Autodesk Inventor part; units mm, degrees
ref_plane "YZ Plane" through (0, 0, 0) normal (1, 0, 0) x (0, 1, 0)
ref_plane "XZ Plane" through (0, 0, 0) normal (0, 1, 0) x (-1, 0, 0)
ref_plane "XY Plane" through (0, 0, 0) normal (0, 0, 1) x (1, 0, 0)
sketch "Sketch1" plane through (0, 0, 0) normal (0, 0, 1) x (1, 0, 0)
  line L0 (-22.1112, 10.3171) -> (130.2888, 10.3171)
  line L1 (130.2888, 10.3171) -> (130.2888, -65.8829)
  line L2 (130.2888, -65.8829) -> (-22.1112, -65.8829)
  line L3 (-22.1112, -65.8829) -> (-22.1112, 10.3171)
  point P0 (0, 0)
  dimension "d0" = 152.4
  dimension "d1" = 76.2
extrude "Extrusion1" add sketch "Sketch1" along normal blind 3.175
sketch "Sketch2" plane through (0, 0, 3.175) normal (0, 0, 1) x (1, 0, 0)
  circle A0 centre (-10.0607, -27.9271) radius 1.85
  circle A1 centre (6.0853, -27.9271) radius 1.85
  circle A2 centre (22.2313, -27.9271) radius 1.85
  circle A3 centre (38.3773, -27.9271) radius 1.85
  circle A4 centre (54.5233, -27.9271) radius 1.85
  circle A5 centre (70.6693, -27.9271) radius 1.85
  circle A6 centre (86.8153, -27.9271) radius 1.85
  point P0 (0, 0)
  dimension "d4" = 3.7
  dimension "d5" = 3.7
  dimension "d6" = 3.7
  dimension "d7" = 12.446
  dimension "d8" = 12.446
  dimension "d9" = 3.7
  dimension "d10" = 12.446
  dimension "d11" = 3.7
  dimension "d12" = 3.7
  dimension "d13" = 3.7
  dimension "d14" = 12.446
  dimension "d15" = 12.446
  dimension "d16" = 12.446
extrude "Extrusion2" add sketch "Sketch2" along normal blind 19.05
sketch "Sketch3" plane through (130.2888, -65.8829, 0) normal (1, 0, 0) x (0, 0, -1)
  line L0 (-11.1509, 83.1688) -> (7.2167, 83.1688)
  line L1 (7.2167, 83.1688) -> (7.2167, -5.5026)
  line L2 (7.2167, -5.5026) -> (-11.1509, -5.5026)
  line L3 (-11.1509, -5.5026) -> (-11.1509, 83.1688)
  point P0 (0, 65.8829)
extrude "Extrusion3" cut sketch "Sketch3" against normal blind 31.75
sketch "Sketch4" plane through (0, 0, 3.175) normal (0, 0, 1) x (1, 0, 0)
  line L0 (43.7795, -14.066) -> (47.6081, -14.066)
  line L1 (47.6081, -14.066) -> (47.6081, -46.0267)
  line L2 (47.6081, -46.0267) -> (43.7795, -46.0267)
  line L3 (43.7795, -46.0267) -> (43.7795, -14.066)
  line L4 (33.3021, -14.066) -> (28.2479, -14.066)
  line L5 (28.2479, -14.066) -> (28.2479, -48.0243)
  line L6 (28.2479, -48.0243) -> (33.3021, -48.0243)
  line L7 (33.3021, -48.0243) -> (33.3021, -14.066)
  line L8 (12.2443, -10.6645) -> (18.3845, -10.6645)
  line L9 (18.3845, -10.6645) -> (18.3845, -49.2753)
  line L10 (18.3845, -49.2753) -> (12.2443, -49.2753)
  line L11 (12.2443, -49.2753) -> (12.2443, -10.6645)
  point P0 (0, 0)
extrude "Extrusion4" [suppressed]
extrude "Extrusion5" [suppressed]
extrude "Extrusion6" add sketch "Sketch4" along normal blind 3.175 contours L0 L1 L2 L3 | L8 L9 L10 L11
extrude "Extrusion7" add sketch "Sketch4" along normal blind 6.35 contours L7 L6 L5 L4
properties part number "gearbasephonecaseFINAL"
Verification items for the finished model (mm, model axes). A direction names the side the tool comes from. Round coordinates to 2 decimals unless told otherwise and drop trailing zeros. Write each loop counter-clockwise with the first axis right and the second up, starting at its lowest first coordinate (ties: lowest second). Pieces come first, ordered by that corner, then holes. Notation, with made-up numbers: (83, 20.5) - (104, 20.5) arc R20 ccw to (104, 26.5) - close; hole circle Ø11 at (-35.5, -13.5). An arc over 180 degrees is marked (long way). Answer as a JSON object with one key per item and string values. Group by question number.
Q1. Section check D-D, the plane x = 87.5. Enter the section's corners in (y, z) (3 decimals), plus the area to 3 significant figures.
Q2. Section check A-A, the plane x = 32. Enter the section's corners in (y, z) (3 decimals).
Q3. Section check B-B, the plane z = 7.75. Enter the section's corners in (x, y).
Q4. Go/stop test with flat-tipped pins: pin 1 Ø12 at (x, y) = (53, -18.5) entering from +Z; pin 2 Ø2 at (y, z) = (-22, 8) entering from -X; pin 3 Ø3 at (y, z) = (-25, 5) entering from +X; pin 4 Ø3 at (x, z) = (-6, 9) entering from +Y. Record where each tip stops, or that it passes through.
Q5. Tool access check on faces 3 (the flat face through (46, -46.027, 5)), 4 (the flat face through (15, -10.664, 5)), 5 (the cylindrical face through (39.37, -29.49, 12.57)), 6 (the flat face through (31, -14.066, 6)), 7 (the flat face through (15, -49.275, 5)). Record the directions out of +Z, -Z, +X, -X, +Y, -Y that give a thin tool (end or side, any length) a straight path to the whole face; none if there is none.
Q6. Mould release check, pull along X, two halves, no side actions. Record for faces 1 (the flat face through (37, -27, 0)), 2 (the flat face through (28.248, -31, 6)): released by +X, released by -X, zero draft, split by the parting line, or undercut.
Q7. Thickness scan on line 1 (Z direction, x = 91, y = -34.5) (3 decimals); line 2 (Z direction, x = 33, y = -34) (3 decimals); line 3 (X direction, y = -34.5, z = 7.75). Record the ranges inside material, lowest first.
Found:
{
 "1": {"outline": "(-65.883, 0) - (10.317, 0) - (10.317, 3.175) - (-26.208, 3.175) - (-26.208, 22.225) - (-29.646, 22.225) - (-29.646, 3.175) - (-65.883, 3.175) - close", "area": "307 mm^2"},
 "2": {"outline": "(-65.883, 0) - (10.317, 0) - (10.317, 3.175) - (-14.066, 3.175) - (-14.066, 9.525) - (-48.024, 9.525) - (-48.024, 3.175) - (-65.883, 3.175) - close"},
 "3": {"outline": "circle Ø3.7 at (-10.06, -27.93); circle Ø3.7 at (6.09, -27.93); circle Ø3.7 at (22.23, -27.93); (28.25, -48.02) - (33.3, -48.02) - (33.3, -14.07) - (28.25, -14.07) - close; circle Ø3.7 at (38.38, -27.93); circle Ø3.7 at (54.52, -27.93); circle Ø3.7 at (70.67, -27.93); circle Ø3.7 at (86.82, -27.93)"},
 "4": {"pin 1": "stops at z = 6.35", "pin 2": "stops at x = 28.25", "pin 3": "stops at x = 87.99", "pin 4": "passes through"},
 "5": {"face 3": "+Z, +X, -Y", "face 4": "+Z, +X, -X, +Y", "face 5": "+Z", "face 6": "+Z, +X, +Y", "face 7": "+Z, +X, -X, -Y"},
 "6": {"face 1": "zero draft", "face 2": "undercut"},
 "7": {"line 1": "z = 0 to 3.175", "line 2": "z = 0 to 9.525", "line 3": "x = 28.25 to 33.3"}
}
